Check sheet for the drawn part. Datum: minimum x, y, z corner. Units: mm. A direction names the side the tool comes from. Give positions to 0.01 mm unless a question says otherwise; leave off trailing zeros. Write each loop counter-clockwise with the first axis right and the second up, starting at its lowest first coordinate (ties: lowest second). Pieces come first, ordered by that corner, then holes. Notation, with made-up numbers: (61.25, 42) -> (108.25, 42) arc R10 ccw to (108.25, 49) -> close; hole circle Ø11 at (89, 43). An arc over 180 degrees is marked (long way). Answer as CSV lines item,"result". Start each with the question number.
1) Sectioned sample at C-C on x = 9. Record the cut outline in (y, z) (1 decimal).
2) Material ranges on L1, parallel to Y at x = 6, z = 9; L2, parallel to Z at x = 11, y = 4.5; L3, parallel to Y at x = 7.5, z = 13 (1 decimal), recorded low to high.
3) Gauge pin test, flat ends, axial feed: pin 1 Ø6 at (x, z) = (7, 42) entering from +Y; pin 2 Ø3 at (x, z) = (9, 36.5) entering from -Y; pin 3 Ø1 at (x, z) = (6.5, 8.5) entering from -Y. Record the tip position at first contact, or that the pin passes through.
4) Sectioned sample at D-D on y = 12. Record the cut outline in (x, z) (1 decimal).
5) Sectioned sample at A-A on z = 39.5. Record the cut outline in (x, y).
6) Tool access check on the marked faces 1 and 2. Record the directions out of +Z, -Z, +X, -X, +Y, -Y that give a thin tool (end or side, any length) a straight path to the whole face; none if there is none.
7) Sectioned sample at B-B on z = 54. Record the cut outline in (x, y), and give its area (3 significant figures).
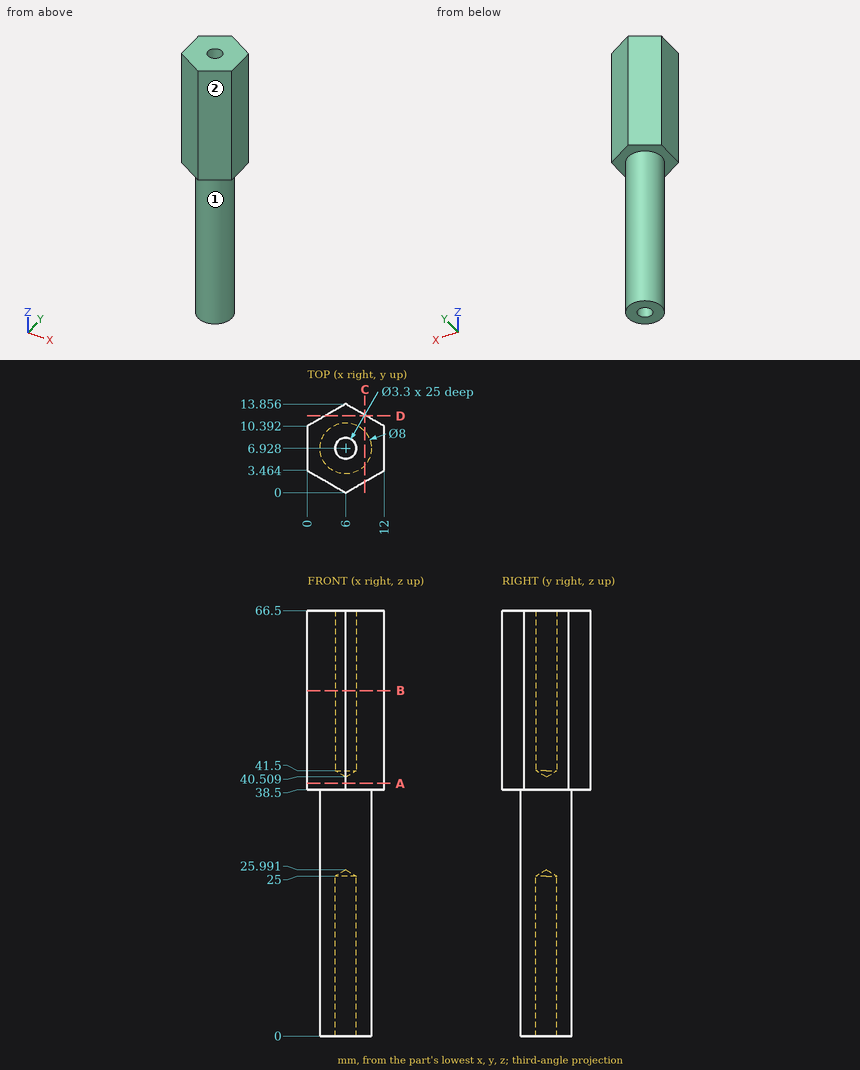
Ans:
1,outline,"(1.7, 38.5) -> (4.3, 38.5) -> (4.3, 0) -> (9.6, 0) -> (9.6, 38.5) -> (12.1, 38.5) -> (12.1, 66.5) -> (1.7, 66.5) -> close"
2,L1,"y = 2.93 to 5.28, 8.58 to 10.93"
2,L2,"z = 38.5 to 66.5"
2,L3,"y = 3.2 to 6.2, 7.6 to 10.6"
3,pin 1,"stops at y = 13.86"
3,pin 2,"stops at y = 3.22"
3,pin 3,"stops at y = 2.93"
4,outline,"(2.8, 38.5) -> (9.2, 38.5) -> (9.2, 66.5) -> (2.8, 66.5) -> close"
5,outline,"(0, 3.46) -> (6, 0) -> (12, 3.46) -> (12, 10.39) -> (6, 13.86) -> (0, 10.39) -> close"
6,face 1,"-Z"
6,face 2,"+Z, -Z, +X, -Y"
7,outline,"(0, 3.46) -> (6, 0) -> (12, 3.46) -> (12, 10.39) -> (6, 13.86) -> (0, 10.39) -> close; hole circle Ø3.3 at (6, 6.93)"
7,area,"116 mm²"
